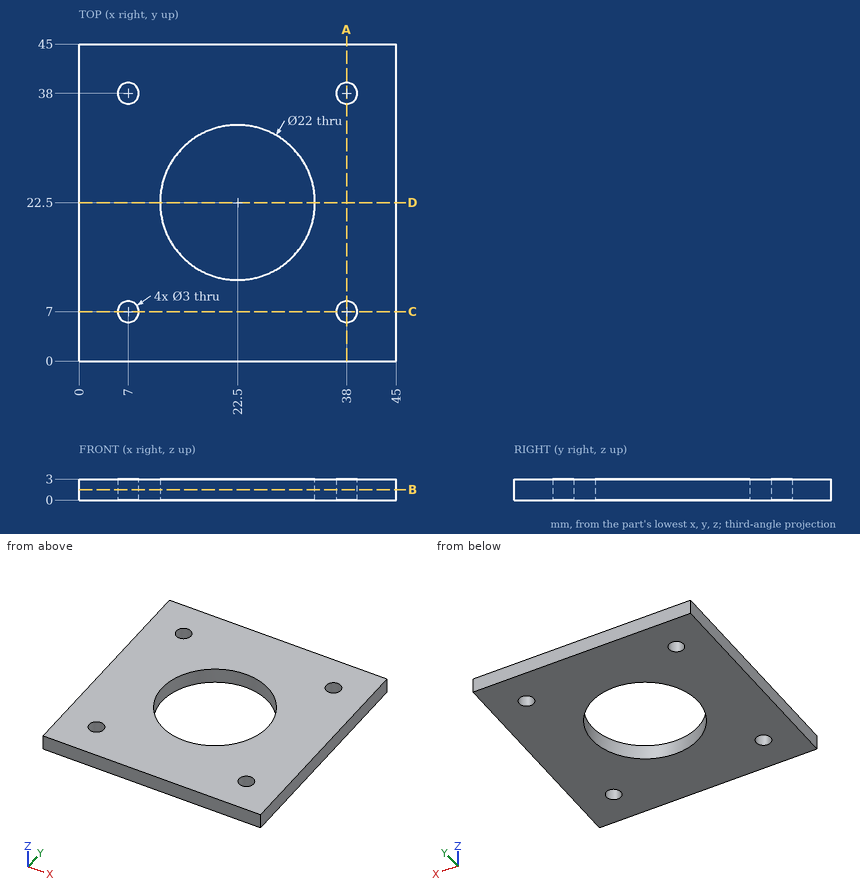
Answer from the drawing. Dimensions are ordinates in mm from the lowest x, y and z of the part. Coordinates: 2 decimals unless noted, no trailing zeros. Order: outer loops, then holes, each group sorted by start corner. A loop starts at its lowest first (then second) coordinate and runs counter-clockwise, first axis right, second up. Notation, with made-up numbers: M -16,65.25 L -7,65.25 A21 ccw -7,78.25 Z; hole C 33.5,-2.5 d1. An arc over 180 degrees is marked long. Put each result on its own line as item: value. Start each with the question number.
Item 1: Section D-D, the plane y = 22.5 is taken. Determine the outline of the cut face in (x, z).
Item 2: Section B-B, the plane z = 1.5 is taken. Determine the outline of the cut face in (x, y).
Item 3: Section A-A, the plane x = 38 is taken. Determine the outline of the cut face in (y, z).
Item 4: Consider probe 1 along Y at (x, z) = (7, 2.2); probe 2 along Y at (x, z) = (37, 1.4). Determine where each line is inside the solid, lowest interval first. Write a range as [from, to].
Computed:
1. outline: M 0,0 L 11.5,0 L 11.5,3 L 0,3 Z; M 33.5,0 L 45,0 L 45,3 L 33.5,3 Z
2. outline: M 0,0 L 45,0 L 45,45 L 0,45 Z; hole C 7,7 d3; hole C 7,38 d3; hole C 22.5,22.5 d22; hole C 38,7 d3; hole C 38,38 d3
3. outline: M 0,0 L 5.5,0 L 5.5,3 L 0,3 Z; M 8.5,0 L 36.5,0 L 36.5,3 L 8.5,3 Z; M 39.5,0 L 45,0 L 45,3 L 39.5,3 Z
4. probe 1: y = [0, 5.5], [8.5, 36.5], [39.5, 45]
4. probe 2: y = [0, 5.88], [8.12, 36.88], [39.12, 45]
